Model file for the job. Use its own axes, mm. Round coordinates to 2 decimals unless told otherwise and drop trailing zeros. Order: outer loops, then holes, each group sorted by start corner. A loop starts at its lowest first (then second) coordinate and runs counter-clockwise, first axis right, second up. Notation, with made-up numbers: (-30.5, -30.5) - (5.5, -30.5) arc R23 ccw to (5.5, -9.5) - close; hole circle Ø11 at (47, 6.25). An arc over 180 degrees is marked (long way). Write item = value, one per line.
```python
from build123d import *

# Parameters (mm, degrees)
SKETCH1_W               = 220
SKETCH1_H               = 180
BOSS_EXTRUDE1_DEPTH     = 3.175
FILLET1_R               = 5
SKETCH2_R               = 50
CUT_EXTRUDE1_DEPTH      = 10
SKETCH5_R               = 1.6
CUT_EXTRUDE3_DEPTH      = 10
MIRROR2_COPY_1_SKETCH_R = 1.6
MIRROR2_COPY_1_DEPTH    = 10
SKETCH7_R               = 2.6
CUT_EXTRUDE4_DEPTH      = 10
CUT_EXTRUDE5_DEPTH      = 10
CUT_EXTRUDE6_DEPTH      = 10


with BuildPart() as part:
    # Sketch1 → Boss-Extrude1 (new body)
    with BuildSketch(Plane(origin=(0, 0, 0), x_dir=(1, 0, 0), z_dir=(0, 1, 0))):
        Rectangle(SKETCH1_W, SKETCH1_H)
    extrude(amount=BOSS_EXTRUDE1_DEPTH)

    # Fillet1
    fillet1_edges = [part.edges().sort_by_distance(p)[0] for p in [
        (-110, 1.5875, -90),
        (110, 1.5875, -90),
        (110, 1.5875, 90),
        (-110, 1.5875, 90),
    ]]
    fillet(fillet1_edges, radius=FILLET1_R)

    # Sketch2 → Cut-Extrude1 (cut)
    with BuildSketch(Plane(origin=(0, 3.175, 0), x_dir=(1, 0, 0), z_dir=(0, 1, 0))):
        with Locations(Location((0, 0, 0), (0, 0, 270))):
            Circle(SKETCH2_R)
    extrude(amount=-CUT_EXTRUDE1_DEPTH, mode=Mode.SUBTRACT)

    # Sketch5 → Cut-Extrude3 (cut)
    with BuildSketch(Plane(origin=(0, 3.175, 0), x_dir=(1, 0, 0), z_dir=(0, 1, 0))):
        with Locations(Location((-70, 81, 0), (0, 0, 270))):
            Circle(SKETCH5_R)
        with Locations(Location((-90, 81, 0), (0, 0, 270))):
            Circle(SKETCH5_R)
        with Locations(Location((-101, 70, 0), (0, 0, 270))):
            Circle(SKETCH5_R)
        with Locations(Location((-101, 50, 0), (0, 0, 270))):
            Circle(SKETCH5_R)
    cut_extrude3 = extrude(amount=-CUT_EXTRUDE3_DEPTH, mode=Mode.SUBTRACT)

    # Mirror1: Cut-Extrude3 across plane
    add(cut_extrude3.mirror(Plane(origin=(0, 0, 0), x_dir=(0, 0, 1), z_dir=(1, 0, 0))), mode=Mode.SUBTRACT)

    # Mirror2: Cut-Extrude3 across plane
    add(cut_extrude3.mirror(Plane.XY), mode=Mode.SUBTRACT)

    # Mirror2 copy 1 sketch → Mirror2 copy 1 (cut)
    with BuildSketch(Plane(origin=(0, 3.175, 0), x_dir=(-1, 0, 0), z_dir=(0, 1, 0))):
        with Locations(Location((-70, 81, 0), (0, 0, 270))):
            Circle(MIRROR2_COPY_1_SKETCH_R)
        with Locations(Location((-90, 81, 0), (0, 0, 270))):
            Circle(MIRROR2_COPY_1_SKETCH_R)
        with Locations(Location((-101, 70, 0), (0, 0, 270))):
            Circle(MIRROR2_COPY_1_SKETCH_R)
        with Locations(Location((-101, 50, 0), (0, 0, 270))):
            Circle(MIRROR2_COPY_1_SKETCH_R)
    extrude(amount=-MIRROR2_COPY_1_DEPTH, mode=Mode.SUBTRACT)

    # Sketch7 → Cut-Extrude4 (cut)
    with BuildSketch(Plane(origin=(0, 3.175, 0), x_dir=(1, 0, 0), z_dir=(0, 1, 0))):
        with Locations(Location((-55, 55, 0), (0, 0, 270))):
            Circle(SKETCH7_R)
        with Locations(Location((55, 55, 0), (0, 0, 270))):
            Circle(SKETCH7_R)
        with Locations(Location((55, -55, 0), (0, 0, 270))):
            Circle(SKETCH7_R)
        with Locations(Location((-55, -55, 0), (0, 0, 270))):
            Circle(SKETCH7_R)
    extrude(amount=-CUT_EXTRUDE4_DEPTH, mode=Mode.SUBTRACT)

    # Sketch8 → Cut-Extrude5 (cut)
    with BuildSketch(Plane(origin=(0, 3.175, 0), x_dir=(1, 0, 0), z_dir=(0, 1, 0))):
        with BuildLine():
            Line((-55, 71.6), (-25, 71.6))
            ThreePointArc((-25, 71.6), (-23.4, 70), (-25, 68.4))
            Line((-25, 68.4), (-55, 68.4))
            ThreePointArc((-55, 68.4), (-56.6, 70), (-55, 71.6))
        make_face()
        with BuildLine():
            Line((55, 68.4), (25, 68.4))
            ThreePointArc((25, 68.4), (23.4, 70), (25, 71.6))
            Line((25, 71.6), (55, 71.6))
            ThreePointArc((55, 71.6), (56.6, 70), (55, 68.4))
        make_face()
    cut_extrude5 = extrude(amount=-CUT_EXTRUDE5_DEPTH, mode=Mode.SUBTRACT)

    # Mirror3: Cut-Extrude5 across plane
    add(cut_extrude5.mirror(Plane.XY), mode=Mode.SUBTRACT)

    # Sketch10 → Cut-Extrude6 (cut)
    with BuildSketch(Plane(origin=(0, 3.175, 0), x_dir=(1, 0, 0), z_dir=(0, 1, 0))):
        with BuildLine():
            Line((-60, 23.4), (-90, 23.4))
            ThreePointArc((-90, 23.4), (-91.6, 25), (-90, 26.6))
            Line((-90, 26.6), (-60, 26.6))
            ThreePointArc((-60, 26.6), (-58.4, 25), (-60, 23.4))
        make_face()
        with BuildLine():
            Line((-90, -23.4), (-60, -23.4))
            ThreePointArc((-60, -23.4), (-58.4, -25), (-60, -26.6))
            Line((-60, -26.6), (-90, -26.6))
            ThreePointArc((-90, -26.6), (-91.6, -25), (-90, -23.4))
        make_face()
    cut_extrude6 = extrude(amount=-CUT_EXTRUDE6_DEPTH, mode=Mode.SUBTRACT)

    # Mirror4: Cut-Extrude6 across plane
    add(cut_extrude6.mirror(Plane(origin=(0, 0, 0), x_dir=(0, 0, 1), z_dir=(1, 0, 0))), mode=Mode.SUBTRACT)


solid = part.part
```
1) Mould opens along Z. For faces 1 (the face through (-54.9, 1.6, -57.6)), 2 (the face through (-109, 2, 88)), 3 (the face through (-50.4, 3.175, -1.3)) say: +Z half, -Z half, draft (parallel to the pull), parting line (faces both ways), or undercut.
Conclusion:
face_1 = undercut
face_2 = +Z half
face_3 = draft
2) Cut at A-A (x = -30). Write the cut outline in (y, z) (3 decimals), and give its area (3 significant figures).
Conclusion:
outline = (0, -90) - (3.175, -90) - (3.175, -71.6) - (0, -71.6) - close; (0, -68.4) - (3.175, -68.4) - (3.175, -40) - (0, -40) - close; (0, 40) - (3.175, 40) - (3.175, 68.4) - (0, 68.4) - close; (0, 71.6) - (3.175, 71.6) - (3.175, 90) - (0, 90) - close
area = 297 mm^2
3) Cut at D-D (y = 2.15). Give the number of separate pieces and of enclosed holes in the cut face, and give its area (3 significant figures).
Conclusion:
separate_pieces = 1
enclosed_holes = 29
area = 30,700 mm^2
4) Cut at B-B (x = 7). Write the cut outline in (y, z) (3 decimals), and give its area (3 significant figures).
Conclusion:
outline = (0, -90) - (3.175, -90) - (3.175, -49.508) - (0, -49.508) - close; (0, 49.508) - (3.175, 49.508) - (3.175, 90) - (0, 90) - close
area = 257 mm^2
5) Flat gauge pin, fed straight in: pin 1 Ø2.5 at (x, z) = (70, -81) entering from +Y. Where does the tip first touch, or does it go through?
Conclusion:
pin_1 = through
6) Cut at C-C (z = -6.5). Write the cut outline in (x, y) (3 decimals), and give its area (3 significant figures).
Conclusion:
outline = (-110, 0) - (-49.576, 0) - (-49.576, 3.175) - (-110, 3.175) - close; (49.576, 0) - (110, 0) - (110, 3.175) - (49.576, 3.175) - close
area = 384 mm^2
7) Wall check: line 1 along X through (y, z) = (1.9, -55); line 2 along X through (y, z) = (2, -81); line 3 along Z through (x, y) = (88, 0.15). Give the ranges that are in metal, low to high.
Conclusion:
line_1 = -110 to -57.6, -52.4 to 52.4, 57.6 to 110
line_2 = -110 to -91.6, -88.4 to -71.6, -68.4 to 68.4, 71.6 to 88.4, 91.6 to 110
line_3 = -90 to -26.6, -23.4 to 23.4, 26.6 to 90
